```python
from build123d import *

# Parameters (mm, degrees)
EXTRUDE17_DEPTH = 1.6129
SKETCH19_R      = 3.6195
EXTRUDE19_DEPTH = 4.2291
SKETCH20_R      = 0.46355
SKETCH20_R_2    = 1.27
EXTRUDE20_DEPTH = 5.2291
SKETCH21_R      = 2.44475
EXTRUDE21_DEPTH = 1.1557
SKETCH22_R      = 2.286
EXTRUDE22_DEPTH = 2.3368


with BuildPart() as part:
    # Sketch18 → Extrude17 (new body)
    with BuildSketch(Plane(origin=(0, 0, 0), x_dir=(1, 0, 0), z_dir=(0, 1, 0))):
        with BuildLine():
            Line((-14.347205988, 1.923996328), (-2.13741415, 2.921))
            ThreePointArc((-2.13741415, 2.921), (3.6195, 0), (-2.13741415, -2.921))
            Line((-2.13741415, -2.921), (-14.347205988, -1.923996328))
            ThreePointArc((-14.347205988, -1.923996328), (-16.1205, 0), (-14.347205988, 1.923996328))
        make_face()
    extrude(amount=EXTRUDE17_DEPTH)

    # Sketch19 → Extrude19 (add)
    with BuildSketch(Plane(origin=(0, 1.6129, 0), x_dir=(1, 0, 0), z_dir=(0, 1, 0))):
        Circle(SKETCH19_R)
    extrude(amount=-EXTRUDE19_DEPTH)

    # Sketch20 → Extrude20 (cut, through all)
    with BuildSketch(Plane(origin=(0, 1.6129, 0), x_dir=(1, 0, 0), z_dir=(0, 1, 0))):
        with Locations((-14.1901, 0)):
            Circle(SKETCH20_R)
        Circle(SKETCH20_R_2)
        with Locations((-4.6651, 0)):
            Circle(SKETCH20_R)
        with Locations((-6.5701, 0)):
            Circle(SKETCH20_R)
        with Locations((-8.4751, 0)):
            Circle(SKETCH20_R)
        with Locations((-10.3801, 0)):
            Circle(SKETCH20_R)
        with Locations((-12.2851, 0)):
            Circle(SKETCH20_R)
    extrude(amount=-EXTRUDE20_DEPTH, mode=Mode.SUBTRACT)

    # Sketch21 → Extrude21 (cut)
    with BuildSketch(Plane(origin=(0, 1.6129, 0), x_dir=(1, 0, 0), z_dir=(0, 1, 0))):
        Circle(SKETCH21_R)
    extrude(amount=-EXTRUDE21_DEPTH, mode=Mode.SUBTRACT)

    # Sketch22 → Extrude22 (cut)
    with BuildSketch(Plane.XZ.offset(2.6162)):
        Circle(SKETCH22_R)
    extrude(amount=-EXTRUDE22_DEPTH, mode=Mode.SUBTRACT)


solid = part.part
```
For this review, take the finished solid that the model builds, in its own axes (mm). A direction names the side the tool comes from. Give positions to 0.01 mm unless a question says otherwise; leave off trailing zeros. Write each loop counter-clockwise with the first axis right and the second up, starting at its lowest first coordinate (ties: lowest second). Pieces come first, ordered by that corner, then holes. Notation, with made-up numbers: M 19,-31.75 L 36,-31.75 A18 ccw 36,-23.75 Z; hole C 68,30 d11. An arc over 180 degrees is marked long. Answer as a JSON object with one key per item and string values. Group by question number.
Item 1: Consider section A-A on x = 0. Write out the cut boundary in (y, z).
Item 2: Consider section B-B on y = 1.3. Write out the cut boundary in (x, z).
Item 3: For pin 1 Ø3 at (x, z) = (-10, -1.5) entering from -Y; pin 2 Ø1 at (x, y) = (-2, 1) entering from +Z; pin 3 Ø1.5 at (x, y) = (-7, 1) entering from -Z; pin 4 Ø1.4 at (x, z) = (-0.5, 0) entering from -Y, all flat-tipped, find the tip position at first contact; note any pin that passes through.
Item 4: Consider section D-D on y = -2.25. Write out the cut boundary in (x, z).
Item 5: Draft analysis for pull direction X (two halves, no side actions). For faces 1 (the cylindrical face through (-4.223, 0.818, -0.139)), 2 (the cylindrical face through (-16.12, 0.8, 0.04)), 3 (the flat face through (-6, 1.613, 1)), state which applies: +X half, -X half, draft (parallel to the pull), parting line (faces both ways), or undercut.
Item 6: Tool access review of faces 4 (the cylindrical face through (-0.53, 1.043, 2.387)), 5 (the flat face through (-8.16, 0.8, 2.43)), 6 (the cylindrical face through (-0.5, -1.46, -2.23)): name each direction out of +Z, -Z, +X, -X, +Y, -Y from which nothing blocks a thin tool from reaching the whole face with its end or side.
Item 7: Consider section C-C on z = 0. Count the separate pieces of the cut face and the enclosed holes in it, plus the area to 3 significant figures.
Item 8: For probe 1 along Z at (x, y) = (0, -2.1); probe 2 along Z at (x, y) = (0, 0.75); probe 3 along X at (y, z) = (-2.05, -1.5), list the stretches that pass through material, from the lowest coordinate up. Write a range as [from, to].
Check result:
{
 "1": {"outline": "M -2.62,-3.62 L 1.61,-3.62 L 1.61,-2.44 L 0.46,-2.44 L 0.46,-1.27 L -0.28,-1.27 L -0.28,-2.29 L -2.62,-2.29 Z; M -2.62,2.29 L -0.28,2.29 L -0.28,1.27 L 0.46,1.27 L 0.46,2.44 L 1.61,2.44 L 1.61,3.62 L -2.62,3.62 Z"},
 "2": {"outline": "M -14.35,-1.92 L -2.14,-2.92 A3.62 ccw long -2.14,2.92 L -14.35,1.92 A1.93 ccw Z; hole C -14.19,0 d0.93; hole C -12.29,0 d0.93; hole C -10.38,0 d0.93; hole C -8.48,0 d0.93; hole C -6.57,0 d0.93; hole C -4.67,0 d0.93; hole C 0,0 d4.89"},
 "3": {"pin 1": "stops at y = 0", "pin 2": "stops at z = 3.29", "pin 3": "stops at z = -2.59", "pin 4": "passes through"},
 "4": {"outline": "C 0,0 d7.24; hole C 0,0 d4.57"},
 "5": {"face 1": "undercut", "face 2": "-X half", "face 3": "draft"},
 "6": {"face 4": "+Y", "face 5": "+Z, -X, +Y, -Y", "face 6": "-Y"},
 "7": {"separate pieces": "8", "enclosed holes": "0", "area": "23.6 mm^2"},
 "8": {"probe 1": "z = [-3.62, -2.29], [2.29, 3.62]", "probe 2": "z = [-3.62, -2.44], [2.44, 3.62]", "probe 3": "x = [-3.29, -1.73], [1.73, 3.29]"}
}
